Source: three-view drawing plus pictorial views. Frame: mm from the lowest corner of the part. Round coordinates to 2 decimals unless told otherwise and drop trailing zeros. Order: outer loops, then holes, each group sorted by start corner. A loop starts at its lowest first (then second) coordinate and runs counter-clockwise, first axis right, second up. Notation, with made-up numbers: (88.5, 70.5) - (93.5, 70.5) arc R30 ccw to (93.5, 93.5) - close; hole circle Ø11 at (13, 84). An arc over 180 degrees is marked (long way). One line per item, written item: value. Start each with the question number.
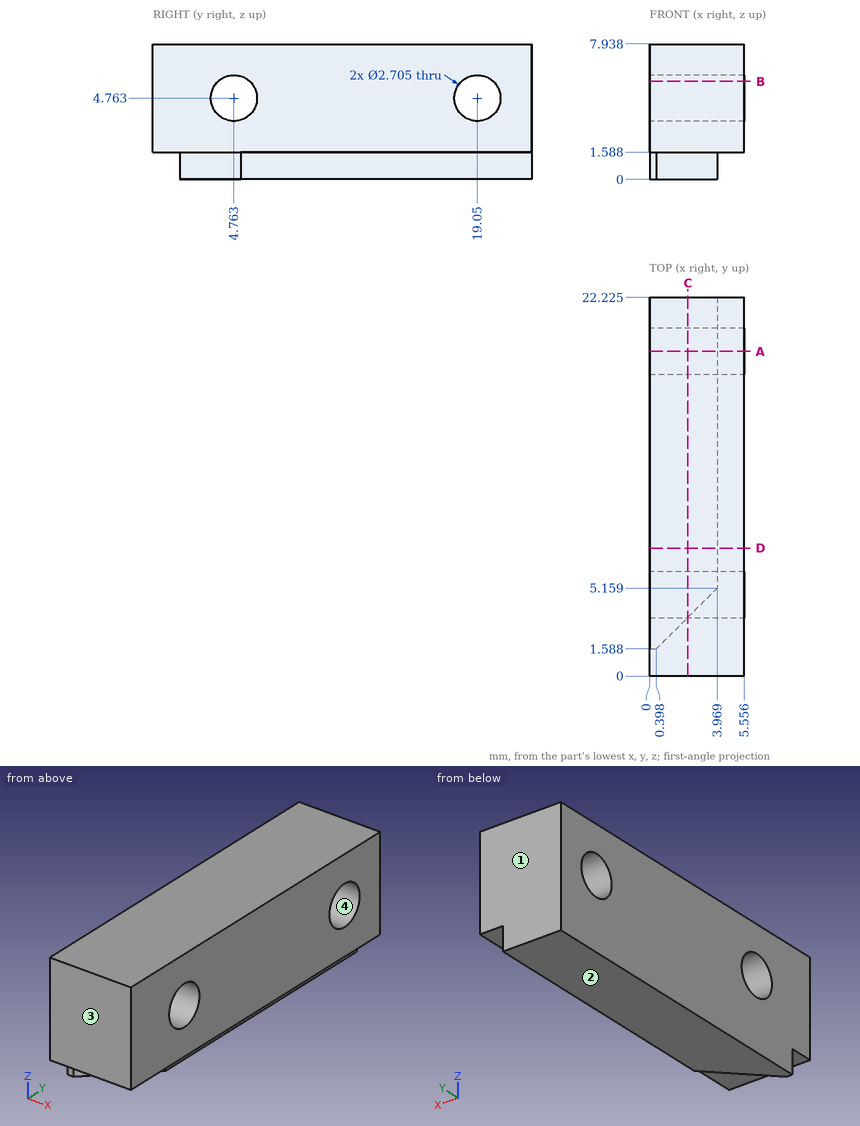
Item 1: Section query C-C on x = 2.25. Give the number of separate pieces and of enclosed holes in the cut face.
Item 2: Pull-direction query (Y, two-part tool) for the marked faces 1, 2, 3 and 4; classes: released by +Y, released by -Y, zero draft, split by the parting line, or undercut.
Item 3: First-contact query: pin 1 Ø0.8 at (y, z) = (11, 1) entering from +X; pin 2 Ø4.5 at (y, z) = (19.05, 4.76) entering from +X. Flat tips, straight axial feed; report the tip coordinate or a pass-through.
Item 4: Section query A-A on y = 19.05. Return loops of the section in (x, z) (1 decimal).
Item 5: Section query B-B on z = 5.75. Return loops of the section in (x, y) (1 decimal), and give its area (3 significant figures).
Item 6: Section query D-D on y = 7.5. Return loops of the section in (x, z), and give its area (3 significant figures).
Item 7: Line query: L1, parallel to Z at x = 3.65, y = 19.05 (1 decimal); L2, parallel to Y at x = 1.6, z = 5.5 (1 decimal); L3, parallel to X at y = 16.5, z = 1. Output: solid intervals per line, ascending.
Geometry results:
1. separate pieces: 1
1. enclosed holes: 2
2. face 1: released by +Y
2. face 2: zero draft
2. face 3: released by -Y
2. face 4: undercut
3. pin 1: stops at x = 3.97
3. pin 2: stops at x = 5.56
4. outline: (0, 0) - (4, 0) - (4, 1.6) - (5.6, 1.6) - (5.6, 3.4) - (0, 3.4) - close; (0, 6.1) - (5.6, 6.1) - (5.6, 7.9) - (0, 7.9) - close
5. outline: (0, 0) - (5.6, 0) - (5.6, 3.8) - (0, 3.8) - close; (0, 5.7) - (5.6, 5.7) - (5.6, 18.1) - (0, 18.1) - close; (0, 20) - (5.6, 20) - (5.6, 22.2) - (0, 22.2) - close
5. area: 103 mm^2
6. outline: (0, 0) - (3.97, 0) - (3.97, 1.59) - (5.56, 1.59) - (5.56, 7.94) - (0, 7.94) - close
6. area: 41.6 mm^2
7. L1: z = 0 to 3.4, 6.1 to 7.9
7. L2: y = 0 to 3.6, 5.9 to 17.9, 20.2 to 22.2
7. L3: x = 0 to 3.97
